```python
from build123d import *

# Parameters (mm, degrees)
SKIZZE1_W                       = 250
SKIZZE1_H                       = 200
AUFSATZ_LINEAR_AUSTRAGEN1_DEPTH = 0.19
SCHNITT_LINEAR_AUSTRAGEN1_DEPTH = 1.19


with BuildPart() as part:
    # Skizze1 → Aufsatz-Linear austragen1 (new body)
    with BuildSketch(Plane.XY):
        with Locations((125, 100)):
            Rectangle(SKIZZE1_W, SKIZZE1_H)
    extrude(amount=AUFSATZ_LINEAR_AUSTRAGEN1_DEPTH)

    # Skizze2 → Schnitt-Linear austragen1 (cut, through all)
    with BuildSketch(Plane.XY.offset(0.19)):
        with BuildLine():
            Line((75, 171), (175, 171))
            ThreePointArc((175, 171), (186, 160), (175, 149))
            Line((175, 149), (75, 149))
            ThreePointArc((75, 149), (64, 160), (75, 171))
        make_face()
        Polygon((220, 200), (250, 170), (250, 200), align=None)
    extrude(amount=-SCHNITT_LINEAR_AUSTRAGEN1_DEPTH, mode=Mode.SUBTRACT)


solid = part.part
```
Verification items for the finished model (mm, model axes). Coordinates: 2 decimals unless noted, no trailing zeros. Write each loop counter-clockwise with the first axis right and the second up, starting at its lowest first coordinate (ties: lowest second). Pieces come first, ordered by that corner, then holes. Notation, with made-up numbers: (-19.5, 9.5) - (24.5, 9.5) arc R13 cw to (24.5, 17.5) - close; hole circle Ø4 at (-0.5, 34). An arc over 180 degrees is marked (long way). One line per question, with ' | ' between items. Start each with the question number.
1. Section check C-C (y = 165.5). Enter the section's corners in (x, z), plus the area to 3 significant figures.
2. Section check A-A (z = 0.1). Enter the section's corners in (x, y), plus the area to 3 significant figures.
3. Section check B-B (x = 122). Enter the section's corners in (y, z).
4. Material ranges on line 1 along Y through (x, z) = (175, 0.1); line 2 along X through (y, z) = (158, 0.1); line 3 along X through (y, z) = (154, 0.15), recorded low to high.
Computed values:
1) outline: (0, 0) - (65.47, 0) - (65.47, 0.19) - (0, 0.19) - close; (184.53, 0) - (250, 0) - (250, 0.19) - (184.53, 0.19) - close | area: 24.9 mm²
2) outline: (0, 0) - (250, 0) - (250, 170) - (220, 200) - (0, 200) - close; hole (75, 149) - (175, 149) arc R11 ccw to (175, 171) - (75, 171) arc R11 ccw to start | area: 47,000 mm²
3) outline: (0, 0) - (149, 0) - (149, 0.19) - (0, 0.19) - close; (171, 0) - (200, 0) - (200, 0.19) - (171, 0.19) - close
4) line 1: 0 to 149, 171 to 200 | line 2: 0 to 64.18, 185.82 to 250 | line 3: 0 to 65.78, 184.22 to 250
